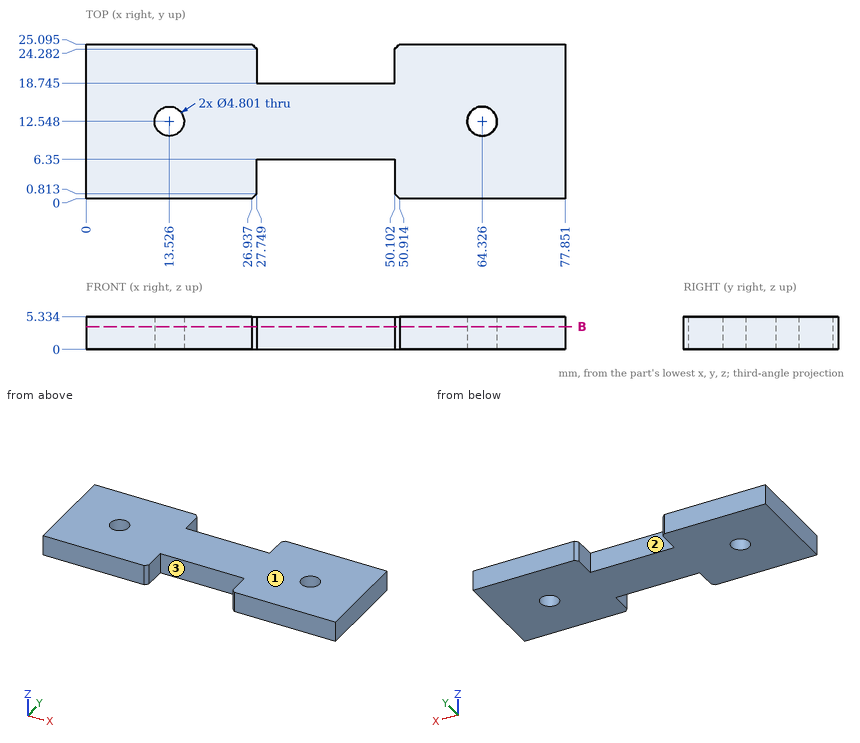
Could you check a few things on this drawing? It's one solid part, dimensions in mm from its lowest x, y, z. A direction names the side the tool comes from. Round coordinates to 2 decimals unless told otherwise and drop trailing zeros.
Q1. Which directions (+Z, -Z, +X, -X, +Y, -Y) give clear straight access to the entire face, cutting with the end or side of a thin tool? Please do the marked faces 1, 2 and 3.
Geometry says:
face 1: +Z, +X, -X, +Y, -Y
face 2: +Z, -Z, +Y
face 3: +Z, -Z, -Y
Q2. Please list where these lines run through material, in increasing order: probe 1 along X at (y, z) = (24, 4.2); probe 2 along X at (y, z) = (13.25, 1.65); probe 3 along Y at (x, z) = (14.5, 2.45) (1 decimal).
Geometry says:
probe 1: x = 0 to 27.75, 50.1 to 77.85
probe 2: x = 0 to 11.23, 15.82 to 62.03, 66.62 to 77.85
probe 3: y = 0 to 10.4, 14.7 to 25.1
Q3. Imagine slicing it at B-B, the plane z = 3.7. State how many separate pieces and enclosed holes the cut face has, then the cut area to 3 significant figures.
Geometry says:
separate pieces: 1
enclosed holes: 2
area: 1,630 mm2
